Input: part model. Units: mm. Frame: model coordinates. A direction names the side the tool comes from. Give positions to 0.01 mm unless a question says otherwise; leave off trailing zeros. Order: outer loops, then holes, each group sorted by start corner. A loop starts at its lowest first (then second) coordinate and runs counter-clockwise, first axis right, second up. Notation, with made-up numbers: (-17.5, 26.25) - (14.5, 26.25) arc R19 ccw to (14.5, 57.25) - close; hole circle Ø6 at (-38, 69.5). An arc over 180 degrees is marked (long way). Answer in a Markdown table with one row per item. Add a question column.
1. Ray query, line 1 (Y direction, x = 0, z = 2.25) (3 decimals); line 2 (Y direction, x = 0, z = 7.2); line 3 (X direction, y = 0, z = 1.5) (1 decimal). Return the intervals inside material, ascending. Write a range as [from, to].
2. Contact query for flat-ended pins moving along their axis: pin 1 (1.9 mm diameter, centred on x = -1, y = 1, fed in from -Z); pin 2 (3 mm diameter, centred on x = 0, y = 0, fed in from -Z) (3 decimals). Output: stop coordinate, or through.
3. Mould query, pull axis X, two halves, no side actions, for faces 5 (the face through (-0.52, -7.56, 2.44)), 6 (the face through (-4.762, 0, 5)), 7 (the face through (-0.69, 3.1, 3.13)). Classes: released by +X, released by -X, zero draft, split by the parting line, or undercut.
4. Access query for faces 1 (the face through (1.4, 1.4, 6.35)), 2 (the face through (-1.1, -4.762, 1.5)), 3 (the face through (0, -8.731, 5)), 4 (the face through (-0.688, 5.545, 1.663)). Directions: +Z, -Z, +X, -X, +Y, -Y. A direction counts if a zero-diameter tool reaches every point of the face in a straight line with its end or side. Return the directions, or none.
5. Section query C-C on z = 8.75. Return loops of the section in (x, y).
```python
from build123d import *

# Parameters (mm, degrees)
F0_W     = 9.525
F0_H     = 9.525
F1_DEPTH = 9.525
F2_R     = 3.175
F3_DEPTH = 6.35
F4_R     = 2.38125
F5_DEPTH = 8.73125
F6_R     = 1.7272
F7_DEPTH = 9.525
F8_R     = 3.175
F9_DEPTH = 6.35


with BuildPart() as f1:
    # F0 (on Top) → F1 (new body)
    with BuildSketch(Plane.XY):
        Rectangle(F0_W, F0_H)
    extrude(amount=F1_DEPTH)

    # F2 (on Front) → F3 (join, symmetric)
    with BuildSketch(Plane.XZ):
        with Locations((0, 4.7625)):
            Circle(F2_R)
    extrude(amount=F3_DEPTH, both=True)

    # F4 (on Front) → F5 (join, symmetric)
    with BuildSketch(Plane.XZ):
        with Locations((0, 4.7625)):
            Circle(F4_R)
    extrude(amount=F5_DEPTH, both=True)

    # F6 (on face) → F7 (cut, through all)
    with BuildSketch(Plane(origin=(0, 0, 0), x_dir=(1, 0, 0), z_dir=(0, 0, -1))):
        Circle(F6_R)
    extrude(amount=-F7_DEPTH, mode=Mode.SUBTRACT)

    # F8 (on face) → F9 (cut)
    with BuildSketch(Plane(origin=(0, 0, 0), x_dir=(1, 0, 0), z_dir=(0, 0, -1))):
        Circle(F8_R)
    extrude(amount=-F9_DEPTH, mode=Mode.SUBTRACT)


solid = f1.part
```
Answer:
| question | item | result |
|---|---|---|
| 1 | line 1 | y = [-6.35, -3.175], [3.175, 6.35] |
| 1 | line 2 | y = [-6.35, -1.73], [1.73, 6.35] |
| 1 | line 3 | x = [-4.8, -3.2], [3.2, 4.8] |
| 2 | pin 1 | stops at z = 6.35 |
| 2 | pin 2 | passes through |
| 3 | face 5 | split by the parting line |
| 3 | face 6 | released by -X |
| 3 | face 7 | undercut |
| 4 | face 1 | -Z |
| 4 | face 2 | -Y |
| 4 | face 3 | +Z, -Z, +X, -X, -Y |
| 4 | face 4 | +Y |
| 5 | outline | (-4.76, -4.76) - (4.76, -4.76) - (4.76, 4.76) - (-4.76, 4.76) - close; hole circle Ø3.45 at (0, 0) |
